Source: three-view drawing plus pictorial views. Frame: mm from the lowest corner of the part. Give positions to 0.01 mm unless a question says otherwise; leave off trailing zeros. Loops run counter-clockwise (first coordinate to the right, second up) from the corner with the lowest first, then second, coordinate; pieces in that order, holes last.
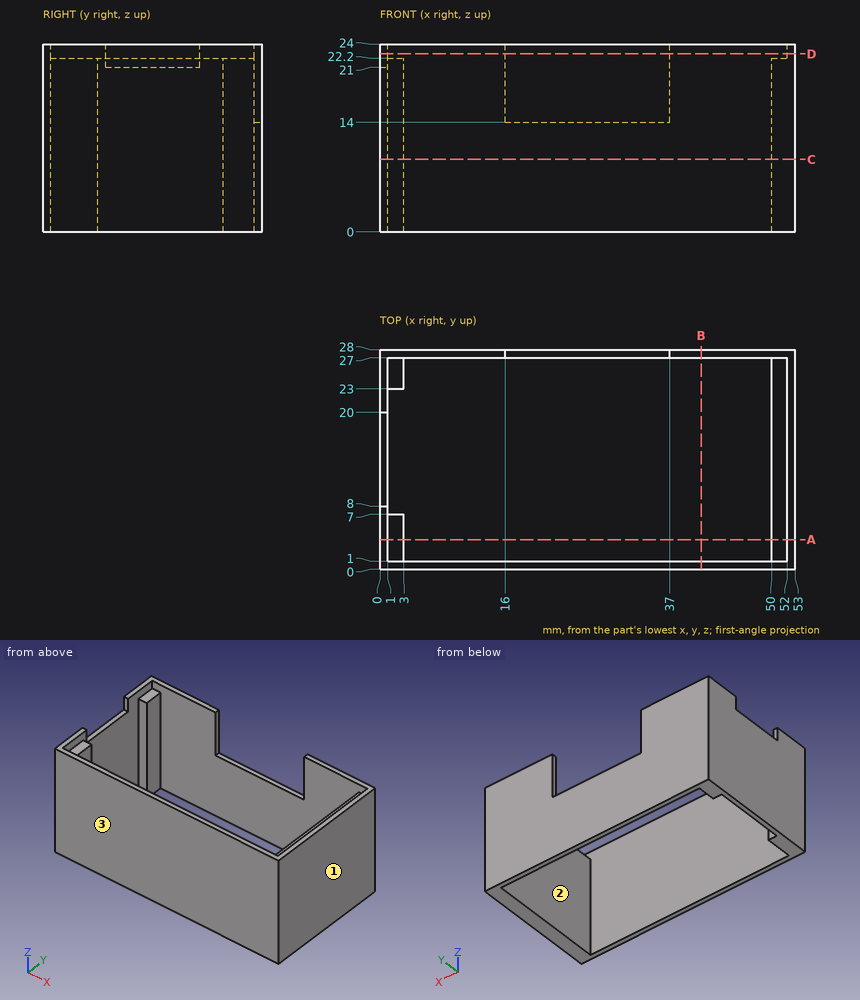
1) Cut plane C-C (z = 9.25). Return loops of the section in (x, y), and give its area (3 significant figures).
Checks:
outline: (0, 0) - (53, 0) - (53, 28) - (0, 28) - close; hole (1, 7) - (3, 7) - (3, 1) - (50, 1) - (50, 27) - (3, 27) - (3, 23) - (1, 23) - close
area: 230 mm2
2) Cut plane A-A (y = 3.75). Return loops of the section in (x, z).
Checks:
outline: (0, 0) - (3, 0) - (3, 22.2) - (1, 22.2) - (1, 24) - (0, 24) - close; (50, 0) - (53, 0) - (53, 24) - (52, 24) - (52, 22.2) - (50, 22.2) - close
3) Contact query for flat-ended pins moving along their axis: P1, Ø0.5, axis at y = 15.5, z = 23, coming from the -X side; P2, Ø5, axis at x = 31, y = 5, coming from the +Z side; P3, Ø2, axis at x = 2.5, y = 24.5, coming from the +Z side. Output: stop coordinate, or through.
Checks:
P1: stops at x = 52
P2: passes through
P3: stops at z = 22.2
4) Ray query, probe 1 along Y at (x, z) = (12, 16.5); probe 2 along X at (y, z) = (18.5, 5); probe 3 along X at (y, z) = (5, 22). Return the intervals inside material, ascending.
Checks:
probe 1: y = 0 to 1, 27 to 28
probe 2: x = 0 to 1, 50 to 53
probe 3: x = 0 to 3, 50 to 53
5) Cut plane D-D (z = 22.75). Return loops of the section in (x, y).
Checks:
outline: (0, 0) - (53, 0) - (53, 28) - (37, 28) - (37, 27) - (52, 27) - (52, 1) - (1, 1) - (1, 8) - (0, 8) - close; (0, 20) - (1, 20) - (1, 27) - (16, 27) - (16, 28) - (0, 28) - close
6) Pull-direction query (Y, two-part tool) for the marked faces 1, 2 and 3; classes: released by +Y, released by -Y, zero draft, split by the parting line, or undercut.
Checks:
face 1: zero draft
face 2: undercut
face 3: released by -Y
7) Cut plane B-B (x = 41). Return loops of the section in (y, z), and give its area (3 significant figures).
Checks:
outline: (0, 0) - (1, 0) - (1, 24) - (0, 24) - close; (27, 0) - (28, 0) - (28, 24) - (27, 24) - close
area: 48.0 mm2
